Verification items for the finished model (mm, model axes). Face numbers are marked on the shaded views. A direction names the side the tool comes from. Coordinates: 2 decimals unless noted, no trailing zeros. Order: outer loops, then holes, each group sorted by start corner. A loop starts at its lowest first (then second) coordinate and runs counter-clockwise, first axis right, second up. Notation, with made-up numbers: (47.5, 72) - (94.5, 72) arc R9 ccw to (94.5, 79) - close; hole circle Ø2 at (50.25, 84.5). An arc over 180 degrees is marked (long way). One line per question, with ' | ' between items. Start each with the question number.
from build123d import *


with BuildPart() as f1:
    # F0 (on Right) → F1 (revolve)
    with BuildSketch(Plane.YZ):
        Polygon((-60.269166, 19.05), (-60.269166, 12.7), (-30.900416, 12.7), (-30.900416, 50.8), (-53.125416, 50.8), (-53.125416, 47.625), (-35.662916, 44.45), (-35.662916, 22.225), align=None)
        Polygon((-30.900416, 50.8), (-30.900416, 12.7), (-1.531666, 12.7), (-1.531666, 19.05), (-26.137916, 22.225), (-26.137916, 44.45), (-8.675416, 47.625), (-8.675416, 50.8), align=None)
    revolve(axis=Axis((0, 4.061773, 0), (0, 1, 0)))


solid = f1.part
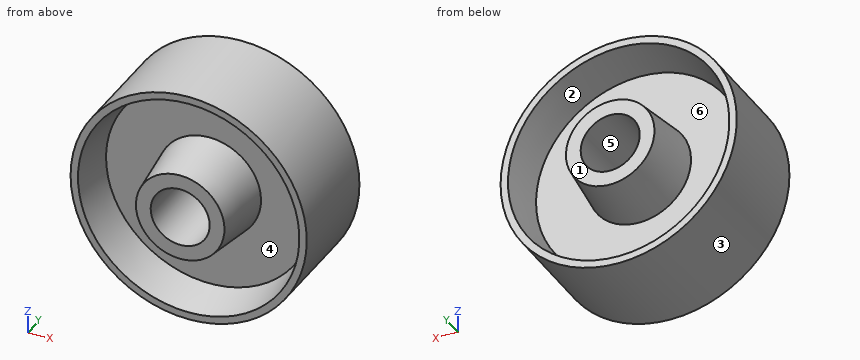
Item 1: Section check D-D (y = -16.5). Record the cut outline in (x, z), then the cut area to 3 significant figures.
Item 2: Gauge pin test, flat ends, axial feed: pin 1 (3 mm diameter, centred on x = 27, z = -24.5, fed in from -Y); pin 2 (1.5 mm diameter, centred on y = -52, z = -15.5, fed in from -X); pin 3 (6 mm diameter, centred on x = 33.5, y = -12.5, fed in from +Z) (3 decimals). Record the tip position at first contact, or that the pin passes through.
Item 3: Set-up check for the marked faces 4, 5 and 6: record each of +Z, -Z, +X, -X, +Y, -Y from which the full face is reachable in a straight line by a thin tool's end or side.
Item 4: Section check B-B (z = 0). Record the cut outline in (x, y) (3 decimals).
Item 5: Section check C-C (y = -32.5). Record the cut outline in (x, z).
Item 6: Mould release check, pull along Z, two halves, no side actions. Record for the marked faces 1, 2 and 3: +Z half, -Z half, draft (parallel to the pull), parting line (faces both ways), or undercut.
Item 7: Section check A-A (x = 0). Record the cut outline in (y, z) (3 decimals), then the cut area to 3 significant figures.
Item 8: Thickness scan on probe 1 along X at (y, z) = (-26, 0); probe 2 along X at (y, z) = (-47, 16); probe 3 along X at (y, z) = (-15, 0). Record the ranges inside material, lowest first. Write a range as from..to.
Completed:
1) outline: circle Ø101.6 at (0, 0); circle Ø41.96 at (0, 0); hole circle Ø92.4 at (0, 0); hole circle Ø25.4 at (0, 0) | area: 2,280 mm^2
2) pin 1: stops at y = -35.66 | pin 2: stops at x = -48.61 | pin 3: stops at z = 40.625
3) face 4: -Y | face 5: +Y, -Y | face 6: +Y
4) outline: (-50.8, -53.125) - (-47.625, -53.125) - (-44.45, -35.663) - (-22.225, -35.663) - (-19.05, -60.269) - (-12.7, -60.269) - (-12.7, -1.532) - (-19.05, -1.532) - (-22.225, -26.138) - (-44.45, -26.138) - (-47.625, -8.675) - (-50.8, -8.675) - close; (12.7, -60.269) - (19.05, -60.269) - (22.225, -35.663) - (44.45, -35.663) - (47.625, -53.125) - (50.8, -53.125) - (50.8, -8.675) - (47.625, -8.675) - (44.45, -26.138) - (22.225, -26.138) - (19.05, -1.532) - (12.7, -1.532) - close
5) outline: circle Ø101.6 at (0, 0); hole circle Ø25.4 at (0, 0)
6) face 1: draft | face 2: undercut | face 3: parting line
7) outline: (-60.269, -19.05) - (-35.663, -22.225) - (-35.663, -44.45) - (-53.125, -47.625) - (-53.125, -50.8) - (-8.675, -50.8) - (-8.675, -47.625) - (-26.138, -44.45) - (-26.138, -22.225) - (-1.532, -19.05) - (-1.532, -12.7) - (-60.269, -12.7) - close; (-60.269, 12.7) - (-1.532, 12.7) - (-1.532, 19.05) - (-26.138, 22.225) - (-26.138, 44.45) - (-8.675, 47.625) - (-8.675, 50.8) - (-53.125, 50.8) - (-53.125, 47.625) - (-35.663, 44.45) - (-35.663, 22.225) - (-60.269, 19.05) - close | area: 1,840 mm^2
8) probe 1: x = -50.8..-44.48, -22.21..-12.7, 12.7..22.21, 44.48..50.8 | probe 2: x = -48.21..-43.67, -13.23..13.23, 43.67..48.21 | probe 3: x = -50.8..-46.48, -20.79..-12.7, 12.7..20.79, 46.48..50.8
